The listing builds one solid part. Answer for the finished solid, in the listing's coordinates (mm). A direction names the side the tool comes from. Give positions to 0.01 mm unless a question says otherwise; leave off trailing zeros. Order: outer loops, then holes, each group sorted by start corner. A loop starts at its lowest first (then second) coordinate and runs counter-clockwise, first axis right, second up. Notation, with made-up numbers: (35, 80.25) - (62, 80.25) arc R12 ccw to (62, 96.25) - close; hole circle Ø7 at (10, -1). An arc over 180 degrees is marked (long way). Use CSV: the item, a comma, the result in double quotes.
```python
from build123d import *

# Parameters (mm, degrees)
ESBO_O4_W                = 7.252623502
ESBO_O4_H                = 0.751020135
CORTE_EXTRUS_O1_DEPTH    = 1
ESBO_O5_W                = 0.6
ESBO_O5_H                = 0.6
RESSALTO_EXTRUS_O1_DEPTH = 27
ESBO_O6_W                = 0.6
ESBO_O6_H                = 0.6
CORTE_EXTRUS_O2_DEPTH    = 1.5
ESBO_O27_R               = 4.624654595
CORTE_EXTRUS_O3_DEPTH    = 24.5


with BuildPart() as part:
    # Esboço1 → Revolução1 (revolve)
    with BuildSketch(Plane(origin=(0, 0, 0), x_dir=(0, 0, -1), z_dir=(1, 0, 0))):
        with BuildLine():
            Line((0, 0), (0, 8.6))
            ThreePointArc((0, 8.6), (1.767766953, 7.867766953), (2.5, 6.1))
            Line((2.5, 6.1), (2.5, 1))
            Line((2.5, 1), (3, 1))
            Line((3, 1), (3, 0))
            Line((3, 0), (0, 0))
        make_face()
    revolve(axis=Axis((0, 0, 0), (0, 1, 0)))

    # Esboço4 → Corte-extrusão1 (cut)
    with BuildSketch(Plane(origin=(0, 0, 0), x_dir=(1, 0, 0), z_dir=(0, 1, 0))):
        with Locations((0, 2.875510068)):
            Rectangle(ESBO_O4_W, ESBO_O4_H)
    extrude(amount=CORTE_EXTRUS_O1_DEPTH, mode=Mode.SUBTRACT)

    # Esboço5 → Ressalto-extrusão1 (add)
    with BuildSketch(Plane.XZ):
        with Locations((0, 1.27)):
            Rectangle(ESBO_O5_W, ESBO_O5_H)
        with Locations((0, -1.27)):
            Rectangle(ESBO_O5_W, ESBO_O5_H)
    extrude(amount=RESSALTO_EXTRUS_O1_DEPTH)

    # Esboço6 → Corte-extrusão2 (cut)
    with BuildSketch(Plane.XZ.offset(27)):
        with Locations((0, -1.27)):
            Rectangle(ESBO_O6_W, ESBO_O6_H)
    extrude(amount=-CORTE_EXTRUS_O2_DEPTH, mode=Mode.SUBTRACT)

    # Esboço27 → Corte-extrusão3 (cut)
    with BuildSketch(Plane.XZ.offset(27)):
        Circle(ESBO_O27_R)
    extrude(amount=-CORTE_EXTRUS_O3_DEPTH, mode=Mode.SUBTRACT)


solid = part.part
```
Item 1: Which of the six approach directions +Z, -Z, +X, -X, +Y, -Y give full straight-line access (tool end or side, diameter ignored) to faces 1 (the face through (2, 1, 2)), 2 (the face through (0, 0.5, -2.5))?
Taken from the geometry:
face 1,"+Y"
face 2,"-Z, +X, -X, +Y, -Y"
Item 2: Each of these flat-tipped pins is pushed along its axis until it touches: pin 1 (0.5 mm diameter, centred on y = -1, z = -1, fed in from -X); pin 2 (1.5 mm diameter, centred on y = -0.5, z = 1, fed in from +X); pin 3 (2 mm diameter, centred on y = 5.5, z = 2, fed in from +X). Where does it stop, or does it pass through?
Taken from the geometry:
pin 1,"x = -0.3"
pin 2,"x = 2.97"
pin 3,"x = 2.29"
Item 3: The part is cut by section C-C (z = 0). Give the vertices of the cut face in (x, y).
Taken from the geometry:
outline,"(-3, 0) - (3, 0) - (3, 1) - (2.5, 1) - (2.5, 6.1) arc R2.5 ccw to (-2.5, 6.1) - (-2.5, 1) - (-3, 1) - close"
Item 4: The part is cut by section B-B (x = 1.2). Give the vertices of the cut face in (y, z).
Taken from the geometry:
outline,"(0, -2.5) - (1, -2.5) - (1, -2.19) - (6.1, -2.19) arc R2.19 ccw to (6.1, 2.19) - (1, 2.19) - (1, 2.75) - (0, 2.75) - close"
Item 5: Find the intervals of material crossed by line 1 along Z through (x, y) = (0.8, 3); line 2 along X through (y, z) = (7.5, -1.75); line 3 along Y through (x, z) = (-2.2, 1.8), in increasing order.
Taken from the geometry:
line 1,"-2.37 to 2.37"
line 2,"-1.11 to 1.11"
line 3,"0 to 1"
Item 6: The part is cut by section D-D (y = 1.5). Give the vertices of the cut face in (x, z).
Taken from the geometry:
outline,"circle Ø5 at (0, 0)"
Item 7: The part is cut by section A-A (y = -1.5). Give the vertices of the cut face in (x, z), and give its area (3 significant figures).
Taken from the geometry:
outline,"(-0.3, -1.57) - (0.3, -1.57) - (0.3, -0.97) - (-0.3, -0.97) - close; (-0.3, 0.97) - (0.3, 0.97) - (0.3, 1.57) - (-0.3, 1.57) - close"
area,"0.720 mm^2"
